For this review, take the finished solid that the model builds, in its own axes (mm). Coordinates: 2 decimals unless noted, no trailing zeros. Order: outer loops, then holes, each group sorted by start corner. A loop starts at its lowest first (then second) coordinate and runs counter-clockwise, first axis right, second up. Notation, with made-up numbers: (-4.5, 34.5) -> (1.5, 34.5) arc R36 ccw to (1.5, 69.5) -> close; hole circle Ø10 at (89.5, -37). An arc over 180 degrees is marked (long way). Answer as a JSON object with one key per item and string values. Group by question number.
1) Wall thickness on L1, parallel to X at y = 2.4, z = 8.25; L2, parallel to Z at x = 42, y = 1.6; L3, parallel to X at y = 1, z = 17.5: over which ranges is each line inside the solid? List them lowest first.
2) Draft analysis for pull direction X (two halves, no side actions). For faces 1 (the flat face through (67.5, 1, 0)), 2 (the flat face through (-1, 3, -14)), 3 (the cylindrical face through (-13.17, 1.52, 17.24)), state which applies: +X half, -X half, draft (parallel to the pull), parting line (faces both ways), or undercut.
3) Add section D-D, the plane x = -51. Write out the cut boundary in (y, z), then the cut area to 3 significant figures.
4) Add section C-C, the plane x = 24. Write out the cut boundary in (y, z).
5) For pin 1 (2 mm diameter, centred on x = 24, z = -17.5, fed in from +Y), flat-tipped, find the tip position at first contact; note if it passes through.
6) Add section B-B, the plane y = 1.65. Count the separate pieces of the cut face and the enclosed holes in it, then the cut area to 3 significant figures.
7) Add section A-A, the plane z = 17.5. Write out the cut boundary in (x, y).
from build123d import *

# Parameters (mm, degrees)
SKETCH1_W           = 135
SKETCH1_H           = 40
SKETCH1_R           = 5
SKETCH1_R_2         = 1.7
SKETCH1_W_2         = 10
SKETCH1_H_2         = 20
BOSS_EXTRUDE1_DEPTH = 3
SKETCH3_R           = 1.2
CUT_EXTRUDE1_DEPTH  = 10


with BuildPart() as part:
    # Sketch1 → Boss-Extrude1 (new body)
    with BuildSketch(Plane(origin=(0, 0, 0), x_dir=(1, 0, 0), z_dir=(0, 1, 0))):
        Rectangle(SKETCH1_W, SKETCH1_H)
        with Locations(Location((-51, 0, 0), (0, 0, 270))):
            Circle(SKETCH1_R, mode=Mode.SUBTRACT)
        with Locations(Location((-60, 8.25, 0), (0, 0, 270))):
            Circle(SKETCH1_R_2, mode=Mode.SUBTRACT)
        with Locations(Location((-42, 8.25, 0), (0, 0, 270))):
            Circle(SKETCH1_R_2, mode=Mode.SUBTRACT)
        with Locations(Location((-42, -8.25, 0), (0, 0, 270))):
            Circle(SKETCH1_R_2, mode=Mode.SUBTRACT)
        with Locations(Location((-60, -8.25, 0), (0, 0, 270))):
            Circle(SKETCH1_R_2, mode=Mode.SUBTRACT)
        with Locations(Location((51, 0, 0), (0, 0, 90))):
            Circle(SKETCH1_R, mode=Mode.SUBTRACT)
        with Locations(Location((42, 8.25, 0), (0, 0, 90))):
            Circle(SKETCH1_R_2, mode=Mode.SUBTRACT)
        with Locations(Location((42, -8.25, 0), (0, 0, 90))):
            Circle(SKETCH1_R_2, mode=Mode.SUBTRACT)
        with Locations(Location((60, -8.25, 0), (0, 0, 90))):
            Circle(SKETCH1_R_2, mode=Mode.SUBTRACT)
        with Locations(Location((60, 8.25, 0), (0, 0, 90))):
            Circle(SKETCH1_R_2, mode=Mode.SUBTRACT)
        Rectangle(SKETCH1_W_2, SKETCH1_H_2, mode=Mode.SUBTRACT)
    extrude(amount=BOSS_EXTRUDE1_DEPTH)

    # Sketch3 → Cut-Extrude1 (cut)
    with BuildSketch(Plane(origin=(0, 3, 0), x_dir=(1, 0, 0), z_dir=(0, 1, 0))):
        with Locations(Location((-12, 17.5, 0), (0, 0, 270))):
            Circle(SKETCH3_R)
        with Locations(Location((-12, -17.5, 0), (0, 0, 270))):
            Circle(SKETCH3_R)
        with Locations(Location((-24, 17.5, 0), (0, 0, 270))):
            Circle(SKETCH3_R)
        with Locations(Location((-24, -17.5, 0), (0, 0, 270))):
            Circle(SKETCH3_R)
        with Locations(Location((24, -17.5, 0), (0, 0, 270))):
            Circle(SKETCH3_R)
        with Locations(Location((24, 17.5, 0), (0, 0, 270))):
            Circle(SKETCH3_R)
        with Locations(Location((12, -17.5, 0), (0, 0, 270))):
            Circle(SKETCH3_R)
        with Locations(Location((12, 17.5, 0), (0, 0, 270))):
            Circle(SKETCH3_R)
    extrude(amount=-CUT_EXTRUDE1_DEPTH, mode=Mode.SUBTRACT)


solid = part.part
Output values:
{
 "1": {"L1": "x = -67.5 to -61.7, -58.3 to -43.7, -40.3 to -5, 5 to 40.3, 43.7 to 58.3, 61.7 to 67.5", "L2": "z = -20 to -9.95, -6.55 to 6.55, 9.95 to 20", "L3": "x = -67.5 to -25.2, -22.8 to -13.2, -10.8 to 10.8, 13.2 to 22.8, 25.2 to 67.5"},
 "2": {"face 1": "+X half", "face 2": "draft", "face 3": "undercut"},
 "3": {"outline": "(0, -20) -> (3, -20) -> (3, -5) -> (0, -5) -> close; (0, 5) -> (3, 5) -> (3, 20) -> (0, 20) -> close", "area": "90.0 mm²"},
 "4": {"outline": "(0, -20) -> (3, -20) -> (3, -18.7) -> (0, -18.7) -> close; (0, -16.3) -> (3, -16.3) -> (3, 16.3) -> (0, 16.3) -> close; (0, 18.7) -> (3, 18.7) -> (3, 20) -> (0, 20) -> close"},
 "5": {"pin 1": "passes through"},
 "6": {"separate pieces": "1", "enclosed holes": "19", "area": "4,930 mm²"},
 "7": {"outline": "(-67.5, 0) -> (-25.2, 0) -> (-25.2, 3) -> (-67.5, 3) -> close; (-22.8, 0) -> (-13.2, 0) -> (-13.2, 3) -> (-22.8, 3) -> close; (-10.8, 0) -> (10.8, 0) -> (10.8, 3) -> (-10.8, 3) -> close; (13.2, 0) -> (22.8, 0) -> (22.8, 3) -> (13.2, 3) -> close; (25.2, 0) -> (67.5, 0) -> (67.5, 3) -> (25.2, 3) -> close"}
}
